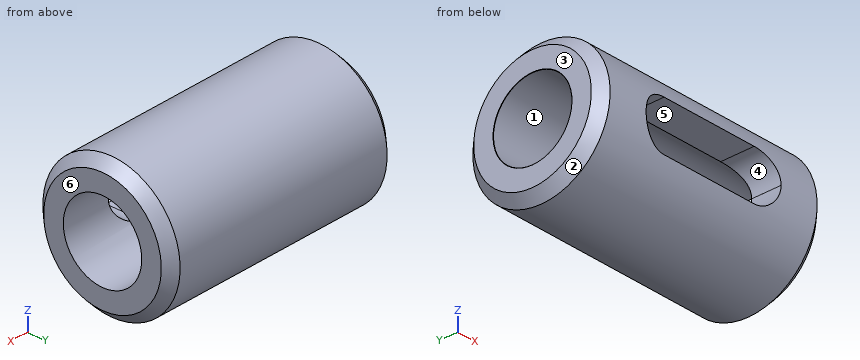
from build123d import *

# Parameters (mm, degrees)
SKETCH_1_W                      = 25
SKETCH_1_H                      = 3
HOLE_WIZARD_8_0_8_1_D           = 8
HOLE_WIZARD_8_0_8_1_DEPTH       = 5
HOLE_WIZARD_8_0_8_1_CSINK_D     = 8.05
HOLE_WIZARD_8_0_8_1_CSINK_ANGLE = 90
HOLE_WIZARD_8_0_8_1_TIP         = 2.403442476
SKETCH_3_W                      = 15
SKETCH_3_H                      = 5
CUT_EXTRUDE_1_DEPTH             = 4
FILLET_1_R                      = 2.5
CHAMFER_1_SIZE                  = 1


with BuildPart() as part:
    # Эскиз1 → Повернуть1 (revolve)
    with BuildSketch(Plane.XY, mode=Mode.PRIVATE) as revolve_1_sk:
        with Locations((0, 5.5)):
            Rectangle(SKETCH_1_W, SKETCH_1_H)
    revolve(revolve_1_sk.sketch.rotate(Axis((0, 0, 0), (-1, 0, 0)), 90), axis=Axis((0, 0, 0), (-1, 0, 0)))

    # Диаметр отверстия Ø8.0 (8)1
    with Locations(Plane.ZY.offset(12.5)):
        with Locations((0, 0)):
            CounterSinkHole(HOLE_WIZARD_8_0_8_1_D / 2, HOLE_WIZARD_8_0_8_1_CSINK_D / 2, depth=HOLE_WIZARD_8_0_8_1_DEPTH, counter_sink_angle=HOLE_WIZARD_8_0_8_1_CSINK_ANGLE)
            with Locations((0, 0, -(HOLE_WIZARD_8_0_8_1_DEPTH + HOLE_WIZARD_8_0_8_1_TIP / 2))):  # 118° drill point
                Cone(0, HOLE_WIZARD_8_0_8_1_D / 2, HOLE_WIZARD_8_0_8_1_TIP, mode=Mode.SUBTRACT)

    # Эскиз3 → Вырез-Вытянуть1 (cut)
    with BuildSketch(Plane(origin=(0, -7, 0), x_dir=(-1, 0, 0), z_dir=(0, -1, 0))):
        Rectangle(SKETCH_3_W, SKETCH_3_H)
    extrude(amount=-CUT_EXTRUDE_1_DEPTH, mode=Mode.SUBTRACT)

    # Скругление1
    fillet_1_edges = [part.edges().sort_by_distance(p)[0] for p in [
        (-7.5, -4.830423707, 2.5),
        (-7.5, -4.830423707, -2.5),
        (7.5, -4.830423707, 2.5),
        (7.5, -4.830423707, -2.5),
    ]]
    fillet(fillet_1_edges, radius=FILLET_1_R - 0.0001)  # a hair under: the kernel refuses the full size

    # Фаска1
    chamfer_1_edges = [part.edges().sort_by_distance(p)[0] for p in [
        (12.5, 0, 7),
        (-12.5, 0, 7),
    ]]
    chamfer(chamfer_1_edges, length=CHAMFER_1_SIZE)


solid = part.part
Here's how the part is built. I have some questions about the finished solid (model axes, mm). Face numbers are marked on the shaded views. A direction names the side the tool comes from. Give positions to 0.01 mm unless a question says otherwise; leave off trailing zeros. Order: outer loops, then holes, each group sorted by start corner. A loop starts at its lowest first (then second) coordinate and runs counter-clockwise, first axis right, second up. Notation, with made-up numbers: M 48,29 L 89,29 A13 cw 89,33 Z; hole C 82.25,2 d11. An arc over 180 degrees is marked long. Answer as a JSON object with one key per item and string values. Group by question number.
1) Suppose I cut it at B-B, the plane x = 8. Write out the boundary of the cut face in (y, z), plus the area to 3 significant figures.
2) On a 3-axis mill with a long thin cutter (end or side, diameter ignored), from which of +Z, -Z, +X, -X, +Y, -Y can I reach the whole of each face in a straight line? I mean the marked faces 5 and 6. Say none if no direction works.
3) I'm going to push flat-ended pins straight in: pin 1 Ø6 at (x, z) = (5.5, 2.5) entering from -Y; pin 2 Ø4 at (x, y) = (2, -5) entering from -Z; pin 3 Ø6 at (x, y) = (10, 3) entering from -Z; pin 4 Ø2.5 at (x, y) = (-1, -4.5) entering from +Z. Where does each tip first touch, or does it pass through?
4) Suppose I cut it at A-A, the plane y = 0. Write out the boundary of the cut face in (x, z) (3 decimals), plus the area to 3 significant figures.
5) Suppose I cut it at C-C, the plane z = -2. Count the separate pieces of the cut face and the enclosed holes in it, plus the area to 3 significant figures.
6) We'd pull the mould along Z, two halves only. Please class the marked faces 1, 2, 3 and 4: pulls with the +Z half, pulls with the -Z half, needs draft (parallel to the pull), parting line crosses it, or undercut.
7) Suppose I cut it at D-D, the plane x = -3. Write out the boundary of the cut face in (y, z).
8) Please list where these lines run through material, in increasing order: L1, parallel to Z at x = -5.5, y = 2; L2, parallel to Z at x = 6.5, y = 2.75; L3, parallel to Y at x = -10.5, z = 0.25. Write a range as [from, to].
Results found:
{
 "1": {"outline": "C 0,0 d14; hole C 0,0 d8", "area": "104 mm²"},
 "2": {"face 5": "-Y", "face 6": "+Z, -Z, +X, +Y, -Y"},
 "3": {"pin 1": "y = -7", "pin 2": "z = -6.32", "pin 3": "z = -7", "pin 4": "z = 6.2"},
 "4": {"outline": "M -12.5,-6 L -11.5,-7 L 11.5,-7 L 12.5,-6 L 12.5,-4 L -12.475,-4 L -12.5,-4.025 Z; M -12.5,4.025 L -12.475,4 L 12.5,4 L 12.5,6 L 11.5,7 L -11.5,7 L -12.5,6 Z", "area": "148 mm²"},
 "5": {"separate pieces": "3", "enclosed holes": "0", "area": "118 mm²"},
 "6": {"face 1": "undercut", "face 2": "parting line crosses it", "face 3": "needs draft", "face 4": "undercut"},
 "7": {"outline": "M -6.54,-2.5 A7 ccw long -6.54,2.5 L -3.12,2.5 A4 cw long -3.12,-2.5 Z"},
 "8": {"L1": "[-6.71, -3.46], [3.46, 6.71]", "L2": "[-6.44, -2.9], [2.9, 6.44]", "L3": "[-7, -3.99], [3.99, 7]"}
}
